from build123d import *

# Parameters (mm, degrees)
SKETCH1_W                    = 190.5
SKETCH1_H                    = 101.6
BOSS_EXTRUDE1_DEPTH          = 3.175
SKETCH2_R                    = 14.2875
CUT_EXTRUDE1_DEPTH           = 3.175
EDGE_FLANGE1_STRIP_W         = 32.7
EDGE_FLANGE1_STRIP_H         = 3.175
EDGE_FLANGE1_STRIP_CUT_DEPTH = 190.5
EDGE_FLANGE1_DEPTH           = 190.5
SKETCH12_R                   = 9.525
SKETCH12_R_2                 = 2.54
CUT_EXTRUDE2_DEPTH           = 7.62
FILLET1_R                    = 38.1


# Sheet-metal steps are written as plain solids
with BuildPart() as part:
    # Sketch1 → Boss-Extrude1 (new body)
    with BuildSketch(Plane(origin=(0, 0, 0), x_dir=(0, 0, -1), z_dir=(1, 0, 0))):
        Rectangle(SKETCH1_W, SKETCH1_H)
    extrude(amount=BOSS_EXTRUDE1_DEPTH)

    # Sketch2 → Cut-Extrude1 (cut)
    with BuildSketch(Plane(origin=(3.175, 0, 0), x_dir=(0, 0, -1), z_dir=(1, 0, 0))):
        with Locations((0, -25.4)):
            Circle(SKETCH2_R)
    extrude(amount=-CUT_EXTRUDE1_DEPTH, mode=Mode.SUBTRACT)

    # Edge-Flange1 strip (across the edge) → Edge-Flange1 strip cut (cut)
    with BuildSketch(Plane(origin=(0, 50.8, 95.25), x_dir=(0, -1, 0), z_dir=(0, 0, -1))):
        with Locations((-3.175, -1.5875)):
            Rectangle(EDGE_FLANGE1_STRIP_W, EDGE_FLANGE1_STRIP_H)
    extrude(amount=EDGE_FLANGE1_STRIP_CUT_DEPTH, mode=Mode.SUBTRACT)

    # Edge-Flange1 section (across the edge) → Edge-Flange1 (add)
    with BuildSketch(Plane(origin=(0, 50.8, 95.25), x_dir=(0, -1, 0), z_dir=(0, 0, -1))):
        with BuildLine():
            Line((0, 10), (0, 22.225))
            Line((0, 22.225), (3.175, 22.225))
            Line((3.175, 22.225), (3.175, 10))
            ThreePointArc((3.175, 10), (6.103932188, 2.928932188), (13.175, 0))
            Line((13.175, 0), (13.175, -3.175))
            ThreePointArc((13.175, -3.175), (3.858868158, 0.683868158), (0, 10))
        make_face()
    extrude(amount=EDGE_FLANGE1_DEPTH)

    # Sketch12 → Cut-Extrude2 (cut)
    with BuildSketch(Plane(origin=(3.175, 0, 0), x_dir=(0, 0, -1), z_dir=(1, 0, 0))):
        with Locations((-47.963329482, 12.225)):
            Circle(SKETCH12_R)
        with Locations((-26.076658964, 25.11428445)):
            Circle(SKETCH12_R_2)
        with Locations((-69.85, -0.66428445)):
            Circle(SKETCH12_R_2)
        with Locations((47.963329482, 12.225)):
            Circle(SKETCH12_R)
        with Locations((26.076658964, 25.11428445)):
            Circle(SKETCH12_R_2)
        with Locations((69.85, -0.66428445)):
            Circle(SKETCH12_R_2)
    extrude(amount=-CUT_EXTRUDE2_DEPTH, mode=Mode.SUBTRACT)

    # Fillet1
    fillet1_edges = [part.edges().sort_by_distance(p)[0] for p in [
        (1.5875, -50.8, 95.25),
        (1.5875, -50.8, -95.25),
    ]]
    fillet(fillet1_edges, radius=FILLET1_R)


solid = part.part
The listing builds one solid part. Answer for the finished solid, in the listing's coordinates (mm). A direction names the side the tool comes from. Coordinates: 2 decimals unless noted, no trailing zeros. Write each loop counter-clockwise with the first axis right and the second up, starting at its lowest first coordinate (ties: lowest second). Pieces come first, ordered by that corner, then holes. Notation, with made-up numbers: M -37,79.25 L -16,79.25 A12 ccw -16,99.25 Z; hole C 1.25,77.5 d2. An arc over 180 degrees is marked long. Write each question's results on one line, items separated by ' | '.
Item 1: Consider probe 1 along Y at (x, z) = (-13.5, -23) (3 decimals); probe 2 along X at (y, z) = (25.5, 47) (3 decimals); probe 3 along Y at (x, z) = (1.5, 69.85). Determine where each line is inside the solid, lowest interval first. Write a range as [from, to].
Answer below:
probe 1: [47.625, 50.8] | probe 2: [0, 3.175] | probe 3: [-48.62, -3.2], [1.88, 44.05]
Item 2: Given P1, Ø3, axis at x = -4, z = -17, coming from the +Y side; P2, Ø17, axis at y = 12.22, z = -47.96, coming from the -X side; P3, Ø6, axis at y = -0.66, z = 69.85, coming from the -X side; P4, Ø10, axis at x = -14, z = 25.5, coming from the -Y side, each flat-ended and moving along its own axis, determine where each tip first touches the part or whether it passes through.
Answer below:
P1: y = 50.01 | P2: through | P3: x = 0 | P4: y = 47.57
Item 3: Which of the six approach directions +Z, -Z, +X, -X, +Y, -Y give full straight-line access (tool end or side, diameter ignored) to faces 1 (the face through (1.61, -11.234, 1.86)), 2 (the face through (0, -6, 1))?
Answer below:
face 1: +X, -X | face 2: +Z, -Z, -X, -Y
Item 4: For a pull along Y with two mould halves and no side action, classify faces 3 (the face through (-0.582, 46.838, 1.334)), 4 (the face through (1, 26, -95.25)), 5 (the face through (1.61, -39.34, -84.39)), 6 (the face through (1.61, 27.633, -25.746)) as released by +Y, released by -Y, zero draft, split by the parting line, or undercut.
Answer below:
face 3: released by +Y | face 4: zero draft | face 5: released by -Y | face 6: undercut
Item 5: The part is cut by section B-B on y = -25.4. Determine the outline of the cut face in (x, z) (1 decimal), and give its area (3 significant figures).
Answer below:
outline: M 0,-93.1 L 3.2,-93.1 L 3.2,-14.3 L 0,-14.3 Z; M 0,14.3 L 3.2,14.3 L 3.2,93.1 L 0,93.1 Z | area: 500 mm2
Item 6: The part is cut by section C-C on z = -60. Determine the outline of the cut face in (x, y) (3 decimals), and give its area (3 significant figures).
Answer below:
outline: M -22.225,47.625 L -10,47.625 A10 cw 0,37.625 L 0,-50.693 L 3.175,-50.693 L 3.175,37.625 A13.175 ccw -10,50.8 L -22.225,50.8 Z | area: 377 mm2
Item 7: The part is cut by section D-D on x = -16.75. Determine the outline of the cut face in (y, z) (3 decimals), and give its area (3 significant figures).
Answer below:
outline: M 47.625,-95.25 L 50.8,-95.25 L 50.8,95.25 L 47.625,95.25 Z | area: 605 mm2
